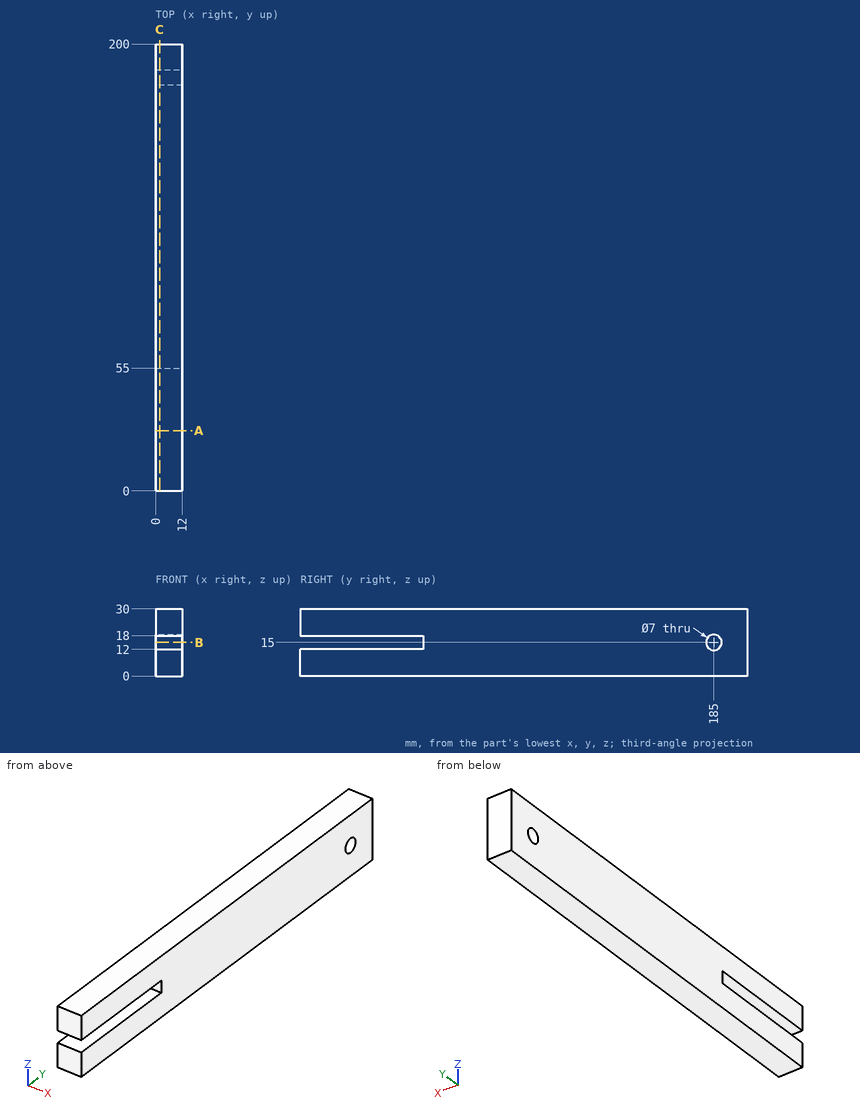
For this review, use the dimensioned drawing (mm, ordinates from the lowest corner) and the shaded views. Coordinates: 2 decimals unless noted, no trailing zeros. Order: outer loops, then holes, each group sorted by start corner. A loop starts at its lowest first (then second) coordinate and runs counter-clockwise, first axis right, second up. Notation, with made-up numbers: (63, 63.5) - (96, 63.5) arc R19 cw to (96, 99.5) - close; hole circle Ø2 at (-21, 55.25). An arc over 180 degrees is marked (long way). Use one line per item in the form item = value.
Q1. Consider section B-B (z = 15). Give the boundary of the cut face in (x, y), then the cut area to 3 significant figures.
Checked values:
outline = (0, 55) - (12, 55) - (12, 181.5) - (0, 181.5) - close; (0, 188.5) - (12, 188.5) - (12, 200) - (0, 200) - close
area = 1,660 mm2
Q2. Consider section A-A (y = 27). Give the boundary of the cut face in (x, z), then the cut area to 3 significant figures.
Checked values:
outline = (0, 0) - (12, 0) - (12, 12) - (0, 12) - close; (0, 18) - (12, 18) - (12, 30) - (0, 30) - close
area = 288 mm2
Q3. Consider section C-C (x = 1.75). Give the boundary of the cut face in (y, z), then the cut area to 3 significant figures.
Checked values:
outline = (0, 0) - (200, 0) - (200, 30) - (0, 30) - (0, 18) - (55, 18) - (55, 12) - (0, 12) - close; hole circle Ø7 at (185, 15)
area = 5,630 mm2
Q4. For probe 1 along Z at (x, y) = (9.25, 185); probe 2 along Y at (x, z) = (4.5, 15.5); probe 3 along Y at (x, z) = (1, 16.5), list the stretches that pass through material, from the lowest coordinate up. Write a range as from..to.
Checked values:
probe_1 = 0..11.5, 18.5..30
probe_2 = 55..181.54, 188.46..200
probe_3 = 55..181.84, 188.16..200
Q5. For P1, Ø5.5, axis at y = 185, z = 15, coming from the -X side; P2, Ø3, axis at x = 6, z = 15.5, coming from the -Y side, all flat-tipped, find the tip position at first contact; note any pin that passes through.
Checked values:
P1 = through
P2 = 55
